Drawing for the job (mm, zero at the part's lowest x, y, z). A direction names the side the tool comes from. Give positions to 0.01 mm unless a question says otherwise; leave off trailing zeros. Order: outer loops, then holes, each group sorted by start corner. A loop starts at its lowest first (then second) coordinate and runs counter-clockwise, first axis right, second up. Notation, with made-up numbers: (-3, 74.5) - (13, 74.5) arc R21 cw to (13, 107.5) - close; hole circle Ø9 at (-7, 37). An arc over 180 degrees is marked (long way). Use a Markdown table: item, result. Add a question column.
(1) Slice it at A-A (y = 48.2). Write the cut outline in (x, z), then the cut area to 3 significant figures.
(2) Wall check: line 1 (X direction, y = 48, z = 17); line 2 (X direction, y = 48, z = 35); line 3 (Z direction, x = 137, y = 39). Give the ranges that are in metal, low to high.
(3) Slice it at B-B (x = 56.5). Write the cut outline in (y, z) (1 decimal).
(4) Slice it at D-D (y = 37). Write the cut outline in (x, z), then the cut area to 3 significant figures.
(5) Which spindle directions (+Z, -Z, +X, -X, +Y, -Y) get a long thin tool onto all of the face, cutting with end or side? Do the marked faces 1 and 2. Say none if no direction does.
(6) Slice it at C-C (z = 22.5). Write the cut outline in (x, y), then the cut area to 3 significant figures.
(7) Mould opens along X. For the marked faces 3, 4, 5 and 6 say: +X half, -X half, draft (parallel to the pull), parting line (faces both ways), or undercut.
(8) Flat gauge pin, fed straight in: pin 1 (15 mm diameter, centred on y = 28.5, z = 45, fed in from +X). Where does the tip first touch, or does it go through?
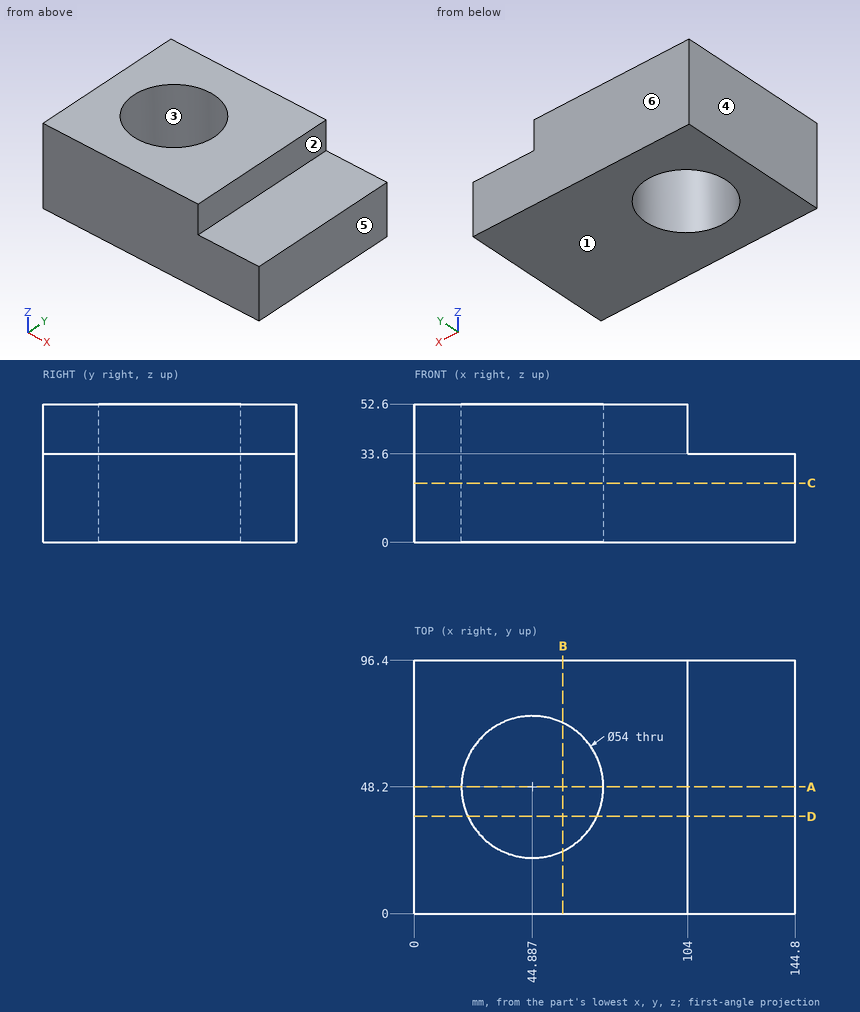
Solution:
| question | item | result |
|---|---|---|
| 1 | outline | (0, 0) - (17.89, 0) - (17.89, 52.6) - (0, 52.6) - close; (71.89, 0) - (144.8, 0) - (144.8, 33.6) - (104, 33.6) - (104, 52.6) - (71.89, 52.6) - close |
| 1 | area | 4,000 mm2 |
| 2 | line 1 | 0 to 17.89, 71.89 to 144.8 |
| 2 | line 2 | 0 to 17.89, 71.89 to 104 |
| 2 | line 3 | 0 to 33.6 |
| 3 | outline | (0, 0) - (23.8, 0) - (23.8, 52.6) - (0, 52.6) - close; (72.6, 0) - (96.4, 0) - (96.4, 52.6) - (72.6, 52.6) - close |
| 4 | outline | (0, 0) - (20.32, 0) - (20.32, 52.6) - (0, 52.6) - close; (69.45, 0) - (144.8, 0) - (144.8, 33.6) - (104, 33.6) - (104, 52.6) - (69.45, 52.6) - close |
| 4 | area | 4,260 mm2 |
| 5 | face 1 | -Z, +X, -X, +Y, -Y |
| 5 | face 2 | +Z, +X, +Y, -Y |
| 6 | outline | (0, 0) - (144.8, 0) - (144.8, 96.4) - (0, 96.4) - close; hole circle Ø54 at (44.89, 48.2) |
| 6 | area | 11,700 mm2 |
| 7 | face 3 | undercut |
| 7 | face 4 | -X half |
| 7 | face 5 | +X half |
| 7 | face 6 | draft |
| 8 | pin 1 | x = 104 |
